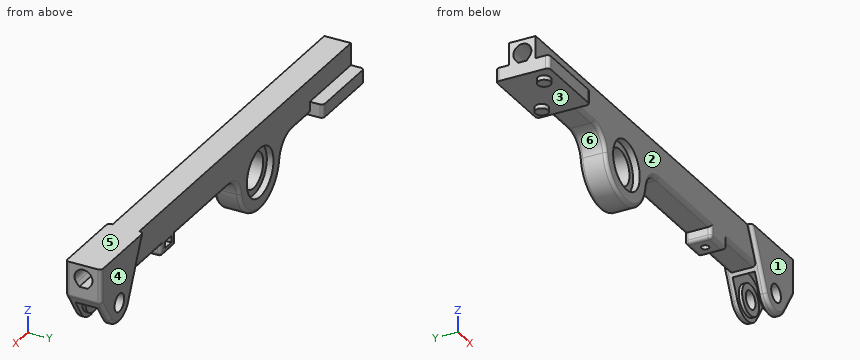
from build123d import *

# Parameters (mm, degrees)
CYLINDER002_R             = 11
CYLINDER002_DEPTH         = 10
CYLINDER003_R             = 8
CYLINDER003_DEPTH         = 28
CYLINDER004_R             = 11
CYLINDER004_DEPTH         = 10
CYLINDER015_R             = 4
CYLINDER015_DEPTH         = 31
CYLINDER017_R             = 7
CYLINDER017_DEPTH         = 2
CYLINDER016_R             = 7
CYLINDER016_DEPTH         = 2
CYLINDER013_R             = 13
CYLINDER013_DEPTH         = 10
CYLINDER023_R             = 1.7
CYLINDER023_DEPTH         = 21
BOX004_W                  = 23
BOX004_H                  = 5.2
BOX004_DEPTH              = 3
PRISM001_DEPTH            = 3
FUSION007_ROLL_ANGLE      = 180
FUSION007_PLACEMENT_ANGLE = 90
EXTRUDE003_DEPTH          = 275
CYLINDER001_R             = 11
CYLINDER001_DEPTH         = 10
BOX001_W                  = 34
BOX001_H                  = 24
BOX001_DEPTH              = 6
EXTRUDE002_DEPTH          = 8
CYLINDER018_R             = 2.9
CYLINDER018_DEPTH         = 2
CYLINDER019_R             = 2.9
CYLINDER019_DEPTH         = 2
EXTRUDE001_DEPTH          = 6
FILLET002_R               = 1.5


with BuildPart() as cilindro002:
    # Cylinder002 → Cylinder002 (new body)
    with BuildSketch(Plane(origin=(83, 3, 55), x_dir=(1, 0, 0), z_dir=(0, 1, 0))):
        Circle(CYLINDER002_R)
    extrude(amount=CYLINDER002_DEPTH)


with BuildPart() as cilindro003:
    # Cylinder003 → Cylinder003 (new body)
    with BuildSketch(Plane(origin=(83, -14, 55), x_dir=(1, 0, 0), z_dir=(0, 1, 0))):
        Circle(CYLINDER003_R)
    extrude(amount=CYLINDER003_DEPTH)


with BuildPart() as cilindro004:
    # Cylinder004 → Cylinder004 (new body)
    with BuildSketch(Plane(origin=(83, -3, 55), x_dir=(1, 0, 0), z_dir=(0, -1, 0))):
        Circle(CYLINDER004_R)
    extrude(amount=CYLINDER004_DEPTH)


with BuildPart() as cilindro015:
    # Cylinder015 → Cylinder015 (new body)
    with BuildSketch(Plane(origin=(203, 15, 55), x_dir=(1, 0, 0), z_dir=(0, -1, 0))):
        Circle(CYLINDER015_R)
    extrude(amount=CYLINDER015_DEPTH)


with BuildPart() as cilindro017:
    # Cylinder017 → Cylinder017 (new body)
    with BuildSketch(Plane(origin=(203, -3.5, 55), x_dir=(1, 0, 0), z_dir=(0, -1, 0))):
        Circle(CYLINDER017_R)
    extrude(amount=CYLINDER017_DEPTH)


with BuildPart() as fusion004:
    # Cylinder016 → Cylinder016 (new body)
    with BuildSketch(Plane(origin=(203, 5.5, 55), x_dir=(1, 0, 0), z_dir=(0, -1, 0))):
        Circle(CYLINDER016_R)
    extrude(amount=CYLINDER016_DEPTH)

    # Fusion004: union Cilindro017
    add(cilindro017.part)


with BuildPart() as cut005:
    # Cylinder013 → Cylinder013 (new body)
    with BuildSketch(Plane(origin=(203, 5, 55), x_dir=(1, 0, 0), z_dir=(0, -1, 0))):
        Circle(CYLINDER013_R)
    extrude(amount=CYLINDER013_DEPTH)

    # Cut005: cut Fusion004
    add(fusion004.part, mode=Mode.SUBTRACT)


with BuildPart() as cilindro023:
    # Cylinder023 → Cylinder023 (new body)
    with BuildSketch(Plane.XY.offset(-6)):
        Circle(CYLINDER023_R)
    extrude(amount=CYLINDER023_DEPTH)


with BuildPart() as cubo004:
    # Box004 → Box004 (new body)
    with BuildSketch(Plane(origin=(0, -2.6, 0), x_dir=(1, 0, 0), z_dir=(0, 0, 1))):
        with Locations((11.5, 2.6)):
            Rectangle(BOX004_W, BOX004_H)
    extrude(amount=BOX004_DEPTH)


with BuildPart() as hueco_tornillo001:
    # Prism001 → Prism001 (new body)
    with BuildSketch(Plane.XY):
        Polygon((3, 0), (1.5, 2.598076), (-1.5, 2.598076), (-3, 0), (-1.5, -2.598076), (1.5, -2.598076), align=None)
    extrude(amount=PRISM001_DEPTH)

    # Fusion007: union Cilindro023, Cubo004
    add(cilindro023.part)
    add(cubo004.part)


with BuildPart() as hueco_tornillo001_1:
    # Fusion007 roll: moved
    add(hueco_tornillo001.part.rotate(Axis((0, 0, 0), (1, 0, 0)), FUSION007_ROLL_ANGLE))


with BuildPart() as hueco_tornillo001_2:
    # Fusion007 placement: moved
    add(hueco_tornillo001_1.part.moved(Location((159, 0, 62))).rotate(Axis((159, 0, 62), (0, 0, 1)), FUSION007_PLACEMENT_ANGLE))


with BuildPart() as extrude003:
    # Sketch003 → Extrude003 (new body)
    with BuildSketch(Plane.YZ):
        with BuildLine():
            ThreePointArc((3.10248, -2.60329), (0, 4.05), (-3.10248, -2.60329))
            Line((-3.10248, -2.60329), (-1.888546, -4.05))
            Line((-1.888546, -4.05), (0, -4.05))
            Line((0, -4.05), (1.888546, -4.05))
            Line((3.10248, -2.60329), (1.888546, -4.05))
        make_face()
    extrude(amount=EXTRUDE003_DEPTH)


with BuildPart() as extrude003_1:
    # Extrude003 placement: moved
    add(extrude003.part.moved(Location((0, 0, 71))))


with BuildPart() as fusion:
    # Cylinder001 → Cylinder001 (new body)
    with BuildSketch(Plane(origin=(83, -3, 55), x_dir=(1, 0, 0), z_dir=(0, -1, 0))):
        Circle(CYLINDER001_R)
    extrude(amount=CYLINDER001_DEPTH)

    # Fusion: union Cilindro002, Cilindro003, Cilindro004, Cilindro015, Cut005, hueco_tornillo001, Extrude003
    add(cilindro002.part)
    add(cilindro003.part)
    add(cilindro004.part)
    add(cilindro015.part)
    add(cut005.part)
    add(hueco_tornillo001_2.part)
    add(extrude003_1.part)


with BuildPart() as cubo001:
    # Box001 → Box001 (new body)
    with BuildSketch(Plane(origin=(8, -12, 61), x_dir=(1, 0, 0), z_dir=(0, 0, 1))):
        with Locations((17, 12)):
            Rectangle(BOX001_W, BOX001_H)
    extrude(amount=BOX001_DEPTH)


with BuildPart() as extrude002:
    # Sketch002 → Extrude002 (new body, symmetric)
    with BuildSketch(Plane.XZ):
        with BuildLine():
            ThreePointArc((194.820389, 51.245808), (202.331926, 46.02483), (210.533656, 50.076178))
            Line((210.533656, 50.076178), (218, 61.5))
            Line((218, 61.5), (218, 77))
            Line((203, 77), (218, 77))
            Line((183, 77), (203, 77))
            Line((183, 77), (194.820389, 51.245808))
        make_face()
    extrude(amount=EXTRUDE002_DEPTH, both=True)


with BuildPart() as cilindro018:
    # Cylinder018 → Cylinder018 (new body)
    with BuildSketch(Plane(origin=(35, 6, 61), x_dir=(1, 0, 0), z_dir=(0, 0, -1))):
        Circle(CYLINDER018_R)
    extrude(amount=CYLINDER018_DEPTH)


with BuildPart() as cilindro019:
    # Cylinder019 → Cylinder019 (new body)
    with BuildSketch(Plane(origin=(15, -6, 61), x_dir=(1, 0, 0), z_dir=(0, 0, -1))):
        Circle(CYLINDER019_R)
    extrude(amount=CYLINDER019_DEPTH)


with BuildPart() as fillet002:
    # Sketch001 → Extrude001 (new body, symmetric)
    with BuildSketch(Plane.XZ):
        with BuildLine():
            Line((8, 77), (218, 77))
            Line((218, 77), (218, 61.5))
            Line((165, 61.5), (218, 61.5))
            Line((165, 56.5), (165, 61.5))
            Line((153, 56.5), (165, 56.5))
            Line((153, 61.5), (153, 56.5))
            Line((109.772187, 61.5), (153, 61.5))
            ThreePointArc((109.772187, 61.5), (103.17533, 59.015416), (99.856562, 52.796296))
            ThreePointArc((66.143438, 52.796296), (83, 38), (99.856562, 52.796296))
            ThreePointArc((66.143438, 52.796296), (62.82467, 59.015416), (56.227813, 61.5))
            Line((8, 61.5), (56.227813, 61.5))
            Line((8, 77), (8, 61.5))
        make_face()
    extrude(amount=EXTRUDE001_DEPTH, both=True)

    # Fusion001: union Cubo001, Extrude002, Cilindro018, Cilindro019
    add(cubo001.part)
    add(extrude002.part)
    add(cilindro018.part)
    add(cilindro019.part)

    # Cut: cut Fusion
    add(fusion.part, mode=Mode.SUBTRACT)

    # Fillet002
    fillet002_edges = [fillet002.edges().sort_by_distance(p)[0] for p in [
        (177.557014, -6, 61.5),
        (49.113906, -6, 61.5),
        (62.82467, -6, 59.015416),
        (159, -6, 56.5),
        (83, -6, 38),
        (153, -6, 59),
        (103.17533, -6, 59.015416),
        (131.386094, -6, 61.5),
        (8, 12, 64),
        (8, -12, 64),
        (188.910194, 8, 64.122904),
        (188.910194, -8, 64.122904),
        (42, 12, 64),
        (42, -12, 64),
        (177.557014, 6, 61.5),
        (49.113906, 6, 61.5),
        (165, 0, 56.5),
        (165, 6, 59),
        (62.82467, 6, 59.015416),
        (153, 0, 56.5),
        (159, 6, 56.5),
        (83, 6, 38),
        (153, 6, 59),
        (103.17533, 6, 59.015416),
        (131.386094, 6, 61.5),
        (202.331926, -8, 46.02483),
        (218, -8, 69.25),
        (214.266828, -8, 55.788089),
        (218, 8, 69.25),
        (218, 0, 61.5),
        (202.331926, 8, 46.02483),
        (214.266828, 8, 55.788089),
    ]]
    fillet(fillet002_edges, radius=FILLET002_R)


solid = fillet002.part
Build history of the part. All positions in model axes, mm. Face numbers are marked on the shaded views. A direction names the side the tool comes from. Coordinates: 2 decimals unless noted, no trailing zeros. Order: outer loops, then holes, each group sorted by start corner. A loop starts at its lowest first (then second) coordinate and runs counter-clockwise, first axis right, second up. Notation, with made-up numbers: (74, 65) - (104, 65) arc R19 ccw to (104, 95) - close; hole circle Ø8 at (46.5, 8). An arc over 180 degrees is marked (long way). Write each question's results on one line, items separated by ' | '. Start each with the question number.
Item 1: Band-saw the part on B-B on x = 35. Write the cut outline in (y, z).
Item 2: Flat gauge pins, fed straight in: pin 1 (8 mm diameter, centred on y = -3.5, z = 44.5, fed in from -X); pin 2 (17.5 mm diameter, centred on x = 207, z = 56, fed in from +Y); pin 3 (17.5 mm diameter, centred on x = 83, z = 55, fed in from +Y). Where does each tip first touch, or does it go through?
Item 3: Mould opens along X. For the marked faces 1 and 2 say: released by +X, released by -X, zero draft, split by the parting line, or undercut.
Item 4: Tool access for the marked faces 3, 4, 5 and 6: list every direction of +Z, -Z, +X, -X, +Y, -Y with a clear straight run to the whole face (end or side of a thin tool).
Item 5: Wall check: probe 1 along Z at (x, y) = (35, 0); probe 2 along Y at (x, z) = (55, 73); probe 3 along X at (y, z) = (0, 58.3). Give the ranges that are in metal, low to high. Write a range as [from, to].
Item 6: Band-saw the part on A-A on x = 119. Write the cut outline in (y, z), and give its area (3 significant figures).
Item 7: Band-saw the part on C-C on x = 201.5. State how many separate pieces and enclosed holes the cut face has, and give its area (3 significant figures).
Numbers:
1) outline: (-12, 61) - (3.1, 61) - (3.1, 59) - (8.9, 59) - (8.9, 61) - (12, 61) - (12, 67) - (6, 67) - (6, 77) - (-6, 77) - (-6, 67) - (-12, 67) - close; hole (-3.1, 68.4) - (-1.89, 66.95) - (1.89, 66.95) - (3.1, 68.4) arc R4.05 ccw (long way) to start
2) pin 1: x = 67.29 | pin 2: y = 8 | pin 3: y = 3
3) face 1: zero draft | face 2: undercut
4) face 3: -Z | face 4: +Z, -Z, +X, +Y | face 5: +Z, +X, -X, +Y, -Y | face 6: -Z, +Y, -Y
5) probe 1: [61, 66.95], [75.05, 77] | probe 2: [-6, -3.52], [3.52, 6] | probe 3: [63.56, 75.71], [90.29, 102.44], [153, 157.3], [160.7, 165], [215.57, 215.91]
6) outline: (-6, 63) arc R1.5 ccw to (-4.5, 61.5) - (4.5, 61.5) arc R1.5 ccw to (6, 63) - (6, 77) - (-6, 77) - close; hole (-3.1, 68.4) - (-1.89, 66.95) - (1.89, 66.95) - (3.1, 68.4) arc R4.05 ccw (long way) to start | area: 133 mm^2
7) separate pieces: 3 | enclosed holes: 0 | area: 201 mm^2
